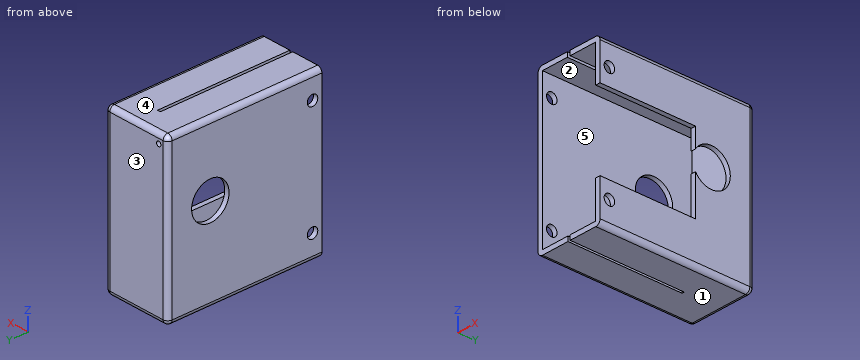
Autodesk Inventor part; units mm, degrees
ref_plane "YZ Plane" through (0, 0, 0) normal (1, 0, 0) x (0, 1, 0)
ref_plane "XZ Plane" through (0, 0, 0) normal (0, 1, 0) x (-1, 0, 0)
ref_plane "XY Plane" through (0, 0, 0) normal (0, 0, 1) x (1, 0, 0)
sketch "Sketch1" plane through (0, 0, 0) normal (0, 1, 0) x (-1, 0, 0)
  line L0 (0, 0) -> (25.4, 0)
  line L1 (25.4, 0) -> (25.4, -101.6)
  line L2 (25.4, -101.6) -> (0, -101.6)
  line L3 (0, -101.6) -> (0, 0)
  line L4 (25.4, 0) -> (31.75, 0)
  line L5 (31.75, 0) -> (31.75, -101.6)
  line L6 (31.75, -101.6) -> (25.4, -101.6)
  line L7 (25.4, -101.6) -> (25.4, 0)
  line L8 (0, -101.6) -> (-6.35, -101.6)
  line L9 (-6.35, -101.6) -> (-6.35, 0)
  line L10 (-6.35, 0) -> (0, 0)
  line L11 (0, 0) -> (0, -101.6)
  line L12 (-6.985, 0.635) -> (32.385, 0.635)
  line L13 (32.385, 0.635) -> (32.385, -102.235)
  line L14 (32.385, -102.235) -> (-6.985, -102.235)
  line L15 (-6.985, -102.235) -> (-6.985, 0.635)
  line L16 (-6.985, 0.635) -> (32.385, -102.235) construction
  line L17 (32.385, 0.635) -> (-6.985, -102.235) construction
  line L18 (-10.16, 3.81) -> (35.56, 3.81)
  line L19 (35.56, 3.81) -> (35.56, -105.41)
  line L20 (35.56, -105.41) -> (-10.16, -105.41)
  line L21 (-10.16, -105.41) -> (-10.16, 3.81)
  line L22 (-10.16, 3.81) -> (35.56, -105.41) construction
  line L23 (35.56, 3.81) -> (-10.16, -105.41) construction
  point P0 (12.7, -50.8)
  dimension "d0" = 25.4
  dimension "d1" = 101.6
  dimension "d2" = 6.35
  dimension "d3" = 6.35
  dimension "d4" = 39.37
  dimension "d5" = 102.87
  dimension "d6" = 45.72
  dimension "d7" = 109.22
extrude "Extrusion1" add sketch "Sketch1" along normal blind 101.6 contours L18 L19 L20 L21
sketch "Sketch2" plane through (10.16, 0, 3.81) normal (1, 0, 0) x (0, 0, -1)
  line L0 (109.22, 0) -> (109.22, 101.6)
  line L1 (109.22, 0) -> (92.71, 0)
  line L2 (92.71, 0) -> (92.71, 6.35)
  line L3 (92.71, 6.35) -> (109.22, 6.35)
  line L4 (109.22, 6.35) -> (109.22, 0)
  line L5 (106.045, 0) -> (3.175, 0)
  line L6 (54.61, 0) -> (54.61, 12.7)
  line L7 (54.61, 12.7) -> (54.61, 63.5)
  line L8 (27.94, 11.43) -> (81.28, 11.43)
  line L9 (81.28, 11.43) -> (81.28, 64.77)
  line L10 (81.28, 64.77) -> (27.94, 64.77)
  line L11 (27.94, 64.77) -> (27.94, 11.43)
  line L12 (27.94, 11.43) -> (81.28, 64.77) construction
  line L13 (81.28, 11.43) -> (27.94, 64.77) construction
  line L14 (27.94, 11.43) -> (81.28, 11.43)
  line L15 (81.28, 11.43) -> (81.28, 0)
  line L16 (81.28, 0) -> (27.94, 0)
  line L17 (27.94, 0) -> (27.94, 11.43)
  line L18 (106.045, 101.6) -> (3.175, 101.6)
  line L19 (54.61, 101.6) -> (54.61, 75.6666)
  line L20 (54.61, 101.6) -> (80.5434, 101.6) construction
  line L21 (54.61, 75.6666) -> (47.5742, 75.6666)
  circle A0 centre (47.5742, 75.6666) radius 12.7
  line L22 (0, 0) -> (0, 101.6)
  line L23 (0, 0) -> (16.51, 0)
  line L24 (16.51, 0) -> (16.51, 6.35)
  line L25 (16.51, 6.35) -> (0, 6.35)
  line L26 (0, 6.35) -> (0, 0)
  point P0 (3.81, 0)
  point P1 (25.4, 6.35)
  point P2 (54.61, 38.1)
  point P3 (41.0508, 64.77)
  point P4 (54.0976, 64.77)
  dimension "d12" = 16.51
  dimension "d13" = 6.35
  dimension "d14" = 12.7
  dimension "d15" = 50.8
  dimension "d16" = 53.34
  dimension "d17" = 53.34
  dimension "d30" = 25.9334
  dimension "d31" = 90
  dimension "d37" = 7.0358
  dimension "d38" = 25.4
  dimension "d48" = 16.51
  dimension "d49" = 6.35
extrude "Extrusion2" cut sketch "Sketch2" against normal blind 3.175 contours L5 L6 L8 L15 | L5 L17 L8 L6 | L8 L11 L10 A0 L9 | A0 L10 picked at (46.2278, 64.3887)
hole "Hole1" at (10.16, 6.35, -88.9) at (10.16, 6.35, -12.7) direction (-1, 0, 0) diameter 7.1374 end through all
sketch "Sketch3" plane through (0, 101.6, 0) normal (0, 1, 0) x (1, 0, 0)
  line L0 (10.16, -3.81) -> (10.16, 105.41)
  line L1 (-35.56, -3.81) -> (10.16, -3.81)
  line L2 (10.16, -3.81) -> (10.16, 105.41)
  line L3 (10.16, 105.41) -> (-35.56, 105.41)
  line L4 (-35.56, 105.41) -> (-35.56, -3.81)
  point P0 (0, 0)
extrude "Extrusion3" add sketch "Sketch3" along normal blind 3.175
fillet "Fillet1" radius 3.175 8 edges at (-12.7, 104.775, 3.81) (10.16, 52.3875, 3.81) (10.16, 104.775, -50.8) (-12.7, 104.775, -105.41) (10.16, 52.3875, -105.41) (-35.56, 104.775, -50.8) (-35.56, 52.3875, 3.81) (-35.56, 52.3875, -105.41)
extrude "Extrusion4" cut sketch "Sketch2" against normal through all contours A0 L10 | L10 A0
sketch "Sketch4" plane through (0, 104.775, 0) normal (0, 1, 0) x (1, 0, 0)
  line L0 (-32.3579, -0.635) -> (-29.1829, -0.635)
  line L1 (-29.1829, -0.635) -> (-29.1829, 2.54)
  line L2 (-29.1829, 2.54) -> (-32.3579, 2.54)
  line L3 (-32.3579, 2.54) -> (-32.3579, -0.635)
  point P0 (0, 0)
  dimension "d39" = 3.175
  dimension "d40" = 3.175
hole "Hole2" at (-29.1829, 104.775, -2.54) direction (0, -1, 0) diameter 3.175 end through all
sketch "Sketch5" plane through (6.985, 0, -105.41) normal (0, 0, -1) x (-1, 0, 0)
  line L0 (-3.175, 64.77) -> (-3.175, 88.3666)
  line L1 (0, 88.3666) -> (0, 64.77)
  line L2 (0, 76.5683) -> (19.685, 76.5683)
  line L3 (39.37, 0) -> (39.37, 101.6)
  line L4 (15.5575, 72.4408) -> (23.8125, 72.4408)
  line L5 (23.8125, 72.4408) -> (23.8125, 80.6958)
  line L6 (23.8125, 80.6958) -> (15.5575, 80.6958)
  line L7 (15.5575, 80.6958) -> (15.5575, 72.4408)
  line L8 (15.5575, 72.4408) -> (23.8125, 80.6958) construction
  line L9 (23.8125, 72.4408) -> (15.5575, 80.6958) construction
  line L10 (19.685, 76.5683) -> (20.4788, 76.5683)
  line L11 (20.4788, 76.5683) -> (20.4788, 77.3621)
  line L12 (20.4788, 77.3621) -> (19.685, 77.3621)
  line L13 (19.685, 77.3621) -> (19.685, 76.5683)
  line L14 (20.4788, 77.3621) -> (18.8913, 77.3621)
  line L15 (18.8913, 77.3621) -> (18.8913, -14.0779)
  line L16 (18.8913, -14.0779) -> (20.4788, -14.0779)
  line L17 (20.4788, -14.0779) -> (20.4788, 77.3621)
  point P0 (6.985, 0)
  dimension "d50" = 19.685
  dimension "d51" = 8.255
  dimension "d52" = 8.255
  dimension "d62" = 0.7937
  dimension "d63" = 0.7937
  dimension "d64" = 1.5875
  dimension "d65" = 91.44
extrude "Extrusion5" cut sketch "Sketch5" against normal blind 6.35 contours L15 L14 L13 L2 | L2 L10 L17 L4 L15 | L13 L12 L11 L10 | L4 L17 L16 L15
sketch "Sketch6" plane through (-32.385, 0, 3.81) normal (0, 0, 1) x (1, 0, 0)
  line L0 (0, 101.6) -> (39.37, 101.6)
  line L1 (19.685, 101.6) -> (19.685, 88.9)
  line L2 (19.685, 88.9) -> (19.685, 89.6938)
  line L3 (19.685, 89.6938) -> (20.4788, 89.6938)
  line L4 (20.4788, 89.6938) -> (18.3833, 89.6938)
  line L5 (18.3833, 89.6938) -> (18.3832, -1.7462)
  line L6 (18.3832, -1.7462) -> (20.4787, -1.7462)
  line L7 (20.4787, -1.7462) -> (20.4788, 89.6938)
  point P0 (32.385, 0)
  dimension "d55" = 12.7
  dimension "d56" = 0.7937
  dimension "d57" = 0.7937
  dimension "d58" = 2.0955
  dimension "d59" = 91.44
extrude "Extrusion6" cut sketch "Sketch6" against normal blind 6.35
properties part number "ThermalOvershield"
CAD build for the part. Positions are in the model's coordinates, mm. Face numbers are marked on the shaded views. A direction names the side the tool comes from. Round coordinates to 2 decimals unless told otherwise and drop trailing zeros. Loops run counter-clockwise (first coordinate to the right, second up) from the corner with the lowest first, then second, coordinate; pieces in that order, holes last. Notation, with made-up numbers: (36, 60.5) - (51, 60.5) arc R27 ccw to (51, 88.5) - close; hole circle Ø6 at (-14.75, 10). An arc over 180 degrees is marked (long way). Return JSON: item names as keys, results as strings. Group by question number.
Q1. Flat gauge pins, fed straight in: pin 1 Ø19.5 at (x, z) = (-8, -25.5) entering from -Y; pin 2 Ø2.5 at (y, z) = (60.5, 2.5) entering from +X; pin 3 Ø2.5 at (y, z) = (61.5, 2) entering from -X. Where does each tip first touch, or does it go through?
Q2. Band-saw the part on C-C on y = 46. Give the cut face in (x, z) (3 decimals).
Q3. Two-plate mould, pull along Z, no slides. Class the marked faces 1, 2 and 3: +Z half, -Z half, draft (parallel to the pull), parting line (faces both ways), or undercut.
Q4. Drill centre lines: line 1 along Z through (x, y) = (-27, 69) (3 decimals); line 2 along X through (y, z) = (96.5, -5.5) (3 decimals); line 3 along Z through (x, y) = (-33.5, 6.35). Where is each one in solid material? Low to high. Write a range as [from, to].
Q5. Band-saw the part on B-B on z = -2.54. Give the cut face in (x, y) (3 decimals).
Q6. Band-saw the part on A-A on z = -88.9. Give the cut face in (x, y) (3 decimals), plus the area to 3 significant figures.
Q7. Tool access for the marked faces 4 and 5: list every direction of +Z, -Z, +X, -X, +Y, -Y with a clear straight run to the whole face (end or side of a thin tool).
Q8. Band-saw the part on D-D on x = -16. Give the cut face in (y, z) (3 decimals).
Solutions:
{
 "1": {"pin 1": "stops at y = 101.6", "pin 2": "stops at x = 10.1", "pin 3": "stops at x = -35.56"},
 "2": {"outline": "(-35.56, -102.235) arc R3.175 ccw to (-32.385, -105.41) - (-13.494, -105.41) - (-13.494, -102.235) - (-32.385, -102.235) - (-32.385, 0.635) - (-14.002, 0.635) - (-14.002, 3.81) - (-32.385, 3.81) arc R3.175 ccw to (-35.56, 0.635) - close; (-11.906, -105.41) - (6.985, -105.41) arc R3.175 ccw to (10.16, -102.235) - (10.16, -77.47) - (6.985, -77.47) - (6.985, -102.235) - (-11.906, -102.235) - close; (-11.906, 0.635) - (6.985, 0.635) - (6.985, -24.13) - (10.16, -24.13) - (10.16, 0.635) arc R3.175 ccw to (6.985, 3.81) - (-11.906, 3.81) - close"},
 "3": {"face 1": "-Z half", "face 2": "undercut", "face 3": "draft"},
 "4": {"line 1": "z = [-105.41, -102.235], [0.635, 3.81]", "line 2": "x = [-35.56, -32.385], [6.985, 10.16]", "line 3": "z = [-105.21, -92.47], [-85.33, -16.27], [-9.13, 3.61]"},
 "5": {"outline": "(-35.56, 0) - (-32.385, 0) - (-32.385, 101.6) - (-30.77, 101.6) - (-30.77, 104.775) - (-32.385, 104.775) arc R3.175 ccw to (-35.56, 101.6) - close; (-27.595, 101.6) - (6.985, 101.6) - (6.985, 0) - (10.16, 0) - (10.16, 101.6) arc R3.175 ccw to (6.985, 104.775) - (-27.595, 104.775) - close"},
 "6": {"outline": "(-35.56, 0) - (-32.385, 0) - (-32.385, 2.781) - (-35.56, 2.781) - close; (-35.56, 9.919) - (-32.385, 9.919) - (-32.385, 101.6) - (6.985, 101.6) - (6.985, 9.919) - (10.16, 9.919) - (10.16, 101.6) arc R3.175 ccw to (6.985, 104.775) - (-32.385, 104.775) arc R3.175 ccw to (-35.56, 101.6) - close; (6.985, 0) - (10.16, 0) - (10.16, 2.781) - (6.985, 2.781) - close", "area": "741 mm^2"},
 "7": {"face 4": "+Z, +X, -X, +Y, -Y", "face 5": "-Y"},
 "8": {"outline": "(0, -105.41) - (101.6, -105.41) arc R3.175 ccw to (104.775, -102.235) - (104.775, 0.635) arc R3.175 ccw to (101.6, 3.81) - (0, 3.81) - (0, 0.635) - (101.6, 0.635) - (101.6, -102.235) - (0, -102.235) - close"}
}
